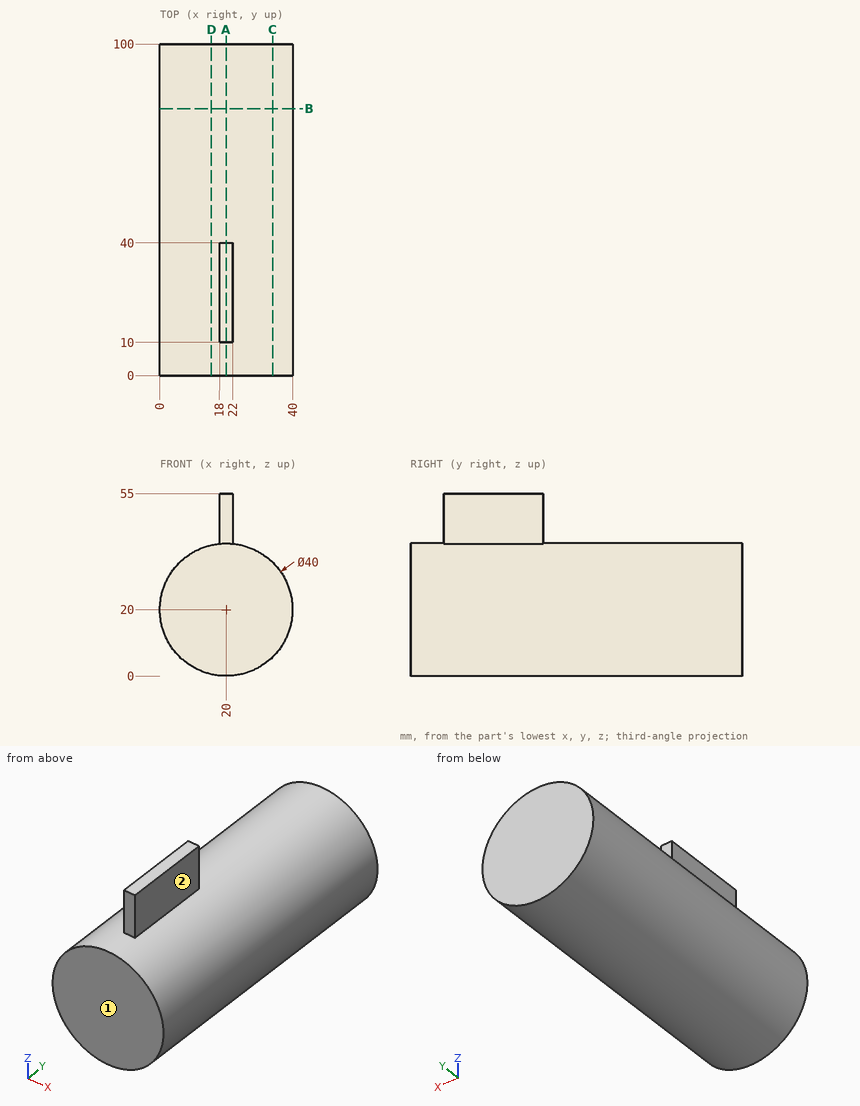
Study the drawing (mm; zero at the part's minimum x, y, z) and answer. A direction names the side the tool comes from. Give positions to 0.01 mm unless a question says otherwise; leave off trailing zeros. Order: outer loops, then holes, each group sorted by start corner. A loop starts at its lowest first (then second) coordinate and runs counter-clockwise, first axis right, second up. Notation, with made-up numbers: (49, -13) -> (94, -13) arc R9 cw to (94, -9) -> close; hole circle Ø1 at (79.5, 39). An arc over 180 degrees is marked (long way). Put each result on its own line as item: value.
Item 1: A cutting plane is placed at A-A on x = 20. Give the vertices of the cut face in (y, z).
Established:
outline: (0, 0) -> (100, 0) -> (100, 40) -> (40, 40) -> (40, 55) -> (10, 55) -> (10, 40) -> (0, 40) -> close
Item 2: Straight lines are drawn through the part: line 1 (X direction, y = 31, z = 19.5); line 2 (X direction, y = 31.5, z = 51); line 3 (Z direction, x = 36, y = 89). For each, find the intervals that lie inside material, in ascending order.
Established:
line 1: x = 0.01 to 39.99
line 2: x = 18 to 22
line 3: z = 8 to 32
Item 3: Given P1, Ø1.5, axis at x = 16, y = 53, coming from the +Z side; P2, Ø7.5, axis at y = 19, z = 45, coming from the +X side; P3, Ø1, axis at x = 30.5, y = 17, coming from the -Z side; P4, Ø10, axis at x = 9.5, z = 22, coming from the -Y side, each flat-ended and moving along its own axis, determine where each tip first touches the part or whether it passes through.
Established:
P1: stops at z = 39.73
P2: stops at x = 22
P3: stops at z = 2.68
P4: stops at y = 0
Item 4: A cutting plane is placed at C-C on x = 34. Give the vertices of the cut face in (y, z), plus the area to 3 significant figures.
Established:
outline: (0, 5.72) -> (100, 5.72) -> (100, 34.28) -> (0, 34.28) -> close
area: 2,860 mm^2
Item 5: For the marked faces 1 and 2, determine the directions among +Z, -Z, +X, -X, +Y, -Y from which every point of the face is accessible in a straight line to the end or side of a thin tool.
Established:
face 1: +Z, -Z, +X, -X, -Y
face 2: +Z, +X, +Y, -Y
Item 6: A cutting plane is placed at B-B on y = 80.5. Give the vertices of the cut face in (x, z), plus the area to 3 significant figures.
Established:
outline: circle Ø40 at (20, 20)
area: 1,260 mm^2
Item 7: A cutting plane is placed at D-D on x = 15.5. Give the vertices of the cut face in (y, z).
Established:
outline: (0, 0.51) -> (100, 0.51) -> (100, 39.49) -> (0, 39.49) -> close
